```python
from build123d import *

# Parameters (mm, degrees)
SKETCH_1_R      = 2.5
SKETCH_1_R_2    = 2
SKETCH_1_W      = 4.718060626
SKETCH_1_H      = 12.511006694
SKETCH_1_W_2    = 4.554527511
SKETCH_1_H_2    = 11.281053154
SKETCH_1_H_3    = 12.511006695
SKETCH_1_H_4    = 11.281053155
EXTRUDE_1_DEPTH = 10


with BuildPart() as part:
    # 草图1 → 凸台-拉伸1 (new body)
    with BuildSketch(Plane.XY):
        with BuildLine():
            ThreePointArc((79.970680431, 2.987579423), (81.435146525, -0.547954483), (84.970680431, -2.012420577))
            Line((84.970680431, -2.012420577), (214.970680431, -2.012420577))
            ThreePointArc((214.970680431, -2.012420577), (218.506214337, -0.547954483), (219.970680431, 2.987579423))
            Line((219.970680431, 2.987579423), (219.970680431, 32.987579423))
            ThreePointArc((219.970680431, 32.987579423), (221.435146525, 36.523113329), (224.970680431, 37.987579423))
            Line((224.970680431, 37.987579423), (294.970680431, 37.987579423))
            ThreePointArc((294.970680431, 37.987579423), (298.506214337, 39.452045517), (299.970680431, 42.987579423))
            Line((299.970680431, 42.987579423), (299.970680431, 252.987579423))
            ThreePointArc((299.970680431, 252.987579423), (298.506214337, 256.523113329), (294.970680431, 257.987579423))
            Line((294.970680431, 257.987579423), (224.970680431, 257.987579423))
            ThreePointArc((224.970680431, 257.987579423), (221.435146525, 259.452045517), (219.970680431, 262.987579423))
            Line((219.970680431, 262.987579423), (219.970680431, 292.987579423))
            ThreePointArc((219.970680431, 292.987579423), (218.506214337, 296.523113329), (214.970680431, 297.987579423))
            Line((214.970680431, 297.987579423), (84.970680431, 297.987579423))
            ThreePointArc((84.970680431, 297.987579423), (81.435146525, 296.523113329), (79.970680431, 292.987579423))
            Line((79.970680431, 292.987579423), (79.970680431, 262.987579423))
            ThreePointArc((79.970680431, 262.987579423), (78.506214337, 259.452045517), (74.970680431, 257.987579423))
            Line((74.970680431, 257.987579423), (4.970680431, 257.987579423))
            ThreePointArc((4.970680431, 257.987579423), (1.435146525, 256.523113329), (-0.029319569, 252.987579423))
            Line((-0.029319569, 252.987579423), (-0.029319569, 42.987579423))
            ThreePointArc((-0.029319569, 42.987579423), (1.435146525, 39.452045517), (4.970680431, 37.987579423))
            Line((4.970680431, 37.987579423), (74.970680431, 37.987579423))
            ThreePointArc((74.970680431, 37.987579423), (78.506214337, 36.523113329), (79.970680431, 32.987579423))
            Line((79.970680431, 32.987579423), (79.970680431, 2.987579423))
        make_face()
        with Locations((9.970680431, 47.987579423)):
            Circle(SKETCH_1_R, mode=Mode.SUBTRACT)
        with BuildLine():
            ThreePointArc((22.970680431, 70.487579423), (24.970680431, 72.487579423), (26.970680431, 70.487579423))
            Line((26.970680431, 70.487579423), (26.970680431, 52.987579423))
            ThreePointArc((26.970680431, 52.987579423), (24.970680431, 50.987579423), (22.970680431, 52.987579423))
            Line((22.970680431, 52.987579423), (22.970680431, 70.487579423))
        make_face(mode=Mode.SUBTRACT)
        with BuildLine():
            ThreePointArc((52.970680431, 70.487579423), (54.970680431, 72.487579423), (56.970680431, 70.487579423))
            Line((56.970680431, 70.487579423), (56.970680431, 52.987579423))
            ThreePointArc((56.970680431, 52.987579423), (54.970680431, 50.987579423), (52.970680431, 52.987579423))
            Line((52.970680431, 52.987579423), (52.970680431, 70.487579423))
        make_face(mode=Mode.SUBTRACT)
        with BuildLine():
            ThreePointArc((76.446824756, 47.714083435), (73.446824756, 44.714083435), (70.446824756, 47.714083435))
            Line((70.446824756, 47.714083435), (70.446824756, 72.714083435))
            ThreePointArc((70.446824756, 72.714083435), (73.446824756, 75.714083435), (76.446824756, 72.714083435))
            Line((76.446824756, 72.714083435), (76.446824756, 47.714083435))
        make_face(mode=Mode.SUBTRACT)
        with Locations((30.470680431, 147.987579423)):
            Circle(SKETCH_1_R, mode=Mode.SUBTRACT)
        with Locations((79.970680431, 98.487579423)):
            Circle(SKETCH_1_R, mode=Mode.SUBTRACT)
        with Locations((129.470680431, 147.987579423)):
            Circle(SKETCH_1_R, mode=Mode.SUBTRACT)
        with BuildLine():
            Line((229.494536105, 72.714083435), (229.494536105, 47.714083435))
            ThreePointArc((229.494536105, 47.714083435), (226.494536105, 44.714083435), (223.494536105, 47.714083435))
            Line((223.494536105, 47.714083435), (223.494536105, 72.714083435))
            ThreePointArc((223.494536105, 72.714083435), (226.494536105, 75.714083435), (229.494536105, 72.714083435))
        make_face(mode=Mode.SUBTRACT)
        with BuildLine():
            ThreePointArc((242.970680431, 70.487579423), (244.970680431, 72.487579423), (246.970680431, 70.487579423))
            Line((246.970680431, 70.487579423), (246.970680431, 52.987579423))
            ThreePointArc((246.970680431, 52.987579423), (244.970680431, 50.987579423), (242.970680431, 52.987579423))
            Line((242.970680431, 52.987579423), (242.970680431, 70.487579423))
        make_face(mode=Mode.SUBTRACT)
        with Locations((289.970680431, 47.987579423)):
            Circle(SKETCH_1_R, mode=Mode.SUBTRACT)
        with BuildLine():
            ThreePointArc((276.970680431, 52.987579423), (274.970680431, 50.987579423), (272.970680431, 52.987579423))
            Line((272.970680431, 52.987579423), (272.970680431, 70.487579423))
            ThreePointArc((272.970680431, 70.487579423), (274.970680431, 72.487579423), (276.970680431, 70.487579423))
            Line((276.970680431, 70.487579423), (276.970680431, 52.987579423))
        make_face(mode=Mode.SUBTRACT)
        with Locations((160.553347356, 126.301390813)):
            Circle(SKETCH_1_R_2, mode=Mode.SUBTRACT)
        with Locations((215.033347356, 126.301390813)):
            Circle(SKETCH_1_R_2, mode=Mode.SUBTRACT)
        with Locations((242.957198236, 106.410275276)):
            Rectangle(SKETCH_1_W, SKETCH_1_H, mode=Mode.SUBTRACT)
        with Locations((289.593492305, 105.795298506)):
            Rectangle(SKETCH_1_W_2, SKETCH_1_H_2, mode=Mode.SUBTRACT)
        with Locations((79.970680431, 197.487579423)):
            Circle(SKETCH_1_R, mode=Mode.SUBTRACT)
        with BuildLine():
            Line((26.970680431, 242.987579423), (26.970680431, 225.487579423))
            ThreePointArc((26.970680431, 225.487579423), (24.970680431, 223.487579423), (22.970680431, 225.487579423))
            Line((22.970680431, 225.487579423), (22.970680431, 242.987579423))
            ThreePointArc((22.970680431, 242.987579423), (24.970680431, 244.987579423), (26.970680431, 242.987579423))
        make_face(mode=Mode.SUBTRACT)
        with Locations((9.970680431, 247.987579423)):
            Circle(SKETCH_1_R, mode=Mode.SUBTRACT)
        with BuildLine():
            Line((56.970680431, 242.987579423), (56.970680431, 225.487579423))
            ThreePointArc((56.970680431, 225.487579423), (54.970680431, 223.487579423), (52.970680431, 225.487579423))
            Line((52.970680431, 225.487579423), (52.970680431, 242.987579423))
            ThreePointArc((52.970680431, 242.987579423), (54.970680431, 244.987579423), (56.970680431, 242.987579423))
        make_face(mode=Mode.SUBTRACT)
        with BuildLine():
            Line((70.446824756, 223.261075411), (70.446824756, 248.261075411))
            ThreePointArc((70.446824756, 248.261075411), (73.446824756, 251.261075411), (76.446824756, 248.261075411))
            Line((76.446824756, 248.261075411), (76.446824756, 223.261075411))
            ThreePointArc((76.446824756, 223.261075411), (73.446824756, 220.261075411), (70.446824756, 223.261075411))
        make_face(mode=Mode.SUBTRACT)
        with Locations((113.606281629, 236.082638095)):
            Circle(SKETCH_1_R_2, mode=Mode.SUBTRACT)
        with Locations((113.606281629, 268.082638095)):
            Circle(SKETCH_1_R_2, mode=Mode.SUBTRACT)
        with Locations((160.553347356, 187.721390813)):
            Circle(SKETCH_1_R_2, mode=Mode.SUBTRACT)
        with Locations((215.033347356, 187.721390813)):
            Circle(SKETCH_1_R_2, mode=Mode.SUBTRACT)
        with Locations((190.106281629, 220.582638095)):
            Circle(SKETCH_1_R_2, mode=Mode.SUBTRACT)
        with Locations((242.957198236, 189.56488357)):
            Rectangle(SKETCH_1_W, SKETCH_1_H_3, mode=Mode.SUBTRACT)
        with Locations((289.593492305, 190.17986034)):
            Rectangle(SKETCH_1_W_2, SKETCH_1_H_4, mode=Mode.SUBTRACT)
        with Locations((189.606281629, 283.582638095)):
            Circle(SKETCH_1_R_2, mode=Mode.SUBTRACT)
        with BuildLine():
            ThreePointArc((223.494536105, 248.261075411), (226.494536105, 251.261075411), (229.494536105, 248.261075411))
            Line((229.494536105, 248.261075411), (229.494536105, 223.261075411))
            ThreePointArc((229.494536105, 223.261075411), (226.494536105, 220.261075411), (223.494536105, 223.261075411))
            Line((223.494536105, 223.261075411), (223.494536105, 248.261075411))
        make_face(mode=Mode.SUBTRACT)
        with BuildLine():
            Line((246.970680431, 242.987579423), (246.970680431, 225.487579423))
            ThreePointArc((246.970680431, 225.487579423), (244.970680431, 223.487579423), (242.970680431, 225.487579423))
            Line((242.970680431, 225.487579423), (242.970680431, 242.987579423))
            ThreePointArc((242.970680431, 242.987579423), (244.970680431, 244.987579423), (246.970680431, 242.987579423))
        make_face(mode=Mode.SUBTRACT)
        with BuildLine():
            Line((272.970680431, 225.487579423), (272.970680431, 242.987579423))
            ThreePointArc((272.970680431, 242.987579423), (274.970680431, 244.987579423), (276.970680431, 242.987579423))
            Line((276.970680431, 242.987579423), (276.970680431, 225.487579423))
            ThreePointArc((276.970680431, 225.487579423), (274.970680431, 223.487579423), (272.970680431, 225.487579423))
        make_face(mode=Mode.SUBTRACT)
        with Locations((289.970680431, 247.987579423)):
            Circle(SKETCH_1_R, mode=Mode.SUBTRACT)
    extrude(amount=EXTRUDE_1_DEPTH)


solid = part.part
```
Here's how the part is built. I have some questions about the finished solid (model axes, mm). A direction names the side the tool comes from. Coordinates: 2 decimals unless noted, no trailing zeros. Loops run counter-clockwise (first coordinate to the right, second up) from the corner with the lowest first, then second, coordinate; pieces in that order, holes last. Notation, with made-up numbers: (55, 16) - (61, 16) arc R34 cw to (61, 46) - close; hole circle Ø11 at (14.25, 31.25). An arc over 180 degrees is marked (long way). Answer as CSV lines item,"result".
Q1. If we section it at A-A, the plane y = 277: Write out the boundary of the cut face in (x, z).
Response:
outline,"(79.97, 0) - (219.97, 0) - (219.97, 10) - (79.97, 10) - close"
Q2. For faces 1 (the face through (148, 150, 10)), 2 (the face through (246.971, 62, 5)), 3 (the face through (259, 37.988, 5)), which set-ups out of +Z, -Z, +X, -X, +Y, -Y let a thin tool reach every point of the face, with its end or its side?
Response:
face 1,"+Z, +X, -X, +Y, -Y"
face 2,"+Z, -Z"
face 3,"+Z, -Z, +X, -Y"
Q3. If we section it at C-C, the plane z = 2.5: Give the number of separate pieces and of enclosed holes in the cut face, and give its area (3 significant figures).
Response:
separate pieces,"1"
enclosed holes,"32"
area,"75,300 mm2"
Q4. If we section it at B-B, the plane x = 234: Write out the boundary of the cut face in (y, z).
Response:
outline,"(37.99, 0) - (257.99, 0) - (257.99, 10) - (37.99, 10) - close"
Q5. We'd pull the mould along Y, two halves only. Please class faces 4 (the face through (151, 297.988, 5)), 5 (the face through (245.316, 189, 5)), 6 (the face through (79.971, 18, 5)): pulls with the +Y half, pulls with the -Y half, needs draft (parallel to the pull), parting line crosses it, or undercut.
Response:
face 4,"pulls with the +Y half"
face 5,"undercut"
face 6,"needs draft"
Q6. If I drill on L1, parallel to X at y = 220.5, z = 9; L2, parallel to Y at x = 130, z = 8.5; L3, parallel to Y at x = 45, z = 7.5, over which ranges is the centre line in solid material (lowest first)? Write a range as [from, to].
Response:
L1,"[-0.03, 72.27], [74.62, 188.11], [192.1, 225.32], [227.67, 299.97]"
L2,"[-2.01, 145.54], [150.43, 297.99]"
L3,"[37.99, 257.99]"
Q7. For pin 1 (5 mm diameter, centred on x = 288.5, z = 6.5, fed in from +Y); pin 2 (3.5 mm diameter, centred on x = 289.5, z = 5, fed in from -Y), each with a flat end and sliding along its axis, tell me the tip position at first contact or that it passes through.
Response:
pin 1,"y = 257.99"
pin 2,"y = 37.99"
